Design review of the part built by this model. Coordinates are the model's own, in mm. Face numbers are marked on the shaded views. A direction names the side the tool comes from. Give positions to 0.01 mm unless a question says otherwise; leave off trailing zeros. Write each loop counter-clockwise with the first axis right and the second up, starting at its lowest first coordinate (ties: lowest second). Pieces come first, ordered by that corner, then holes. Notation, with made-up numbers: (26.25, 11.25) -> (57.25, 11.25) arc R13 cw to (57.25, 27.25) -> close; hole circle Ø11 at (19.5, 45). An arc over 180 degrees is marked (long way). Write each question's results on one line, items separated by ' | '. Start each with the question number.
(1) For the marked faces 1 and 2, list the 3-axis set-ups (+Z, -Z, +X, -X, +Y, -Y) from which the entire face can be reached by the end or side of a thin tool; tool diameter is ignored.
(2) Take a section at A-A (z = 33). State the section outline as (x, y) points, plus the area to 3 significant figures.
(3) To check wall thickness, follow probe 1 along X at (y, z) = (0.25, 43); probe 2 along Y at (x, z) = (-3.25, 60); probe 3 along Y at (x, z) = (4.75, 31.5). State the ranges of each line that lie inside material, in increasing order.
(4) Clearance check with flat-ended pins moving along their axes: pin 1 (1 mm diameter, centred on x = -1, y = 7, fed in from -Z); pin 2 (1 mm diameter, centred on x = 3.5, z = 58, fed in from +Y); pin 3 (4 mm diameter, centred on x = -2, z = 67.5, fed in from -Y). State where each tip first meets the part, or that it passes through.
from build123d import *

# Parameters (mm, degrees)
F2_W     = 25.4
F2_H     = 1.5875
F3_DEPTH = 12.7


with BuildPart() as f1:
    # F0 (on Right) → F1 (revolve)
    with BuildSketch(Plane.YZ):
        Polygon((6.35, 76.2), (0, 76.2), (0, 0), (12.7, 21.997045), (6.35, 21.997045), align=None)
    revolve(axis=Axis((0, 0, 38.1), (0, 0, -1)))

    # F2 (on face) → F3 (cut)
    with BuildSketch(Plane.XY.offset(76.2)):
        Rectangle(F2_W, F2_H)
    extrude(amount=-F3_DEPTH, mode=Mode.SUBTRACT)


solid = f1.part
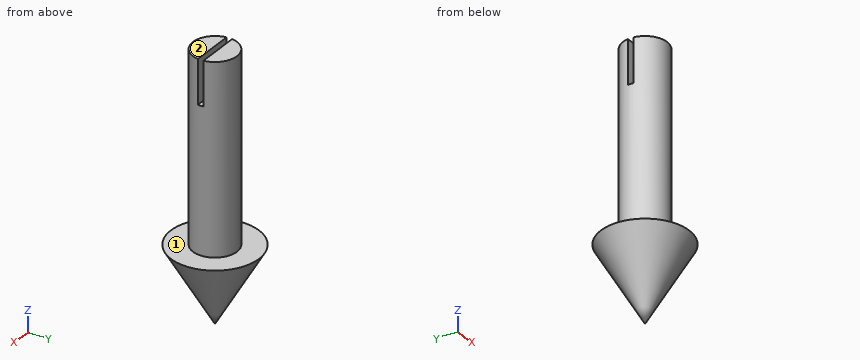
Report:
1) face 1: +Z | face 2: +Z, +X, -X, +Y, -Y
2) outline: circle Ø12.7 at (0, 0) | area: 127 mm2
3) probe 1: -6.35 to 6.35 | probe 2: -5.46 to 5.46 | probe 3: -4.21 to 4.21
4) pin 1: z = 11.38 | pin 2: y = 5.6 | pin 3: y = -6.35
